Work out the finished part from the listing and answer in its coordinate system (mm). A direction names the side the tool comes from. Coordinates: 2 decimals unless noted, no trailing zeros. Order: outer loops, then holes, each group sorted by start corner. A loop starts at its lowest first (then second) coordinate and runs counter-clockwise, first axis right, second up. Notation, with made-up numbers: M 77,8 L 98,8 A28 cw 98,28 Z; hole C 15,55 d8. An arc over 180 degrees is marked long. Use a Markdown table: item, result.
from build123d import *

# Parameters (mm, degrees)
CROQUIS1_W              = 250
CROQUIS1_H              = 100
SALIENTE_EXTRUIR1_DEPTH = 240
CROQUIS1_3_W            = 250
CROQUIS1_3_H            = 100
SALIENTE_EXTRUIR2_DEPTH = 10
REDONDEO2_R             = 60
CROQUIS7_RX             = 76.972297538
CROQUIS7_RY             = 67.204239475
CORTAR_EXTRUIR4_DEPTH   = 143
CROQUIS8_RX             = 76.972297538
CROQUIS8_RY             = 67.204239475
SALIENTE_EXTRUIR3_DEPTH = 5
CROQUIS10_W             = 80
CROQUIS10_H             = 10
SALIENTE_EXTRUIR4_DEPTH = 140
CROQUIS10_4_W           = 60
CROQUIS10_4_H           = 40
SALIENTE_EXTRUIR5_DEPTH = 5
CROQUIS10_7_W           = 10
CROQUIS10_7_H           = 40
SALIENTE_EXTRUIR6_DEPTH = 40
REDONDEO3_R             = 10


with BuildPart() as part:
    # Croquis1 → Saliente-Extruir1 (new body)
    with BuildSketch(Plane(origin=(0, 0, 0), x_dir=(1, 0, 0), z_dir=(0, 1, 0))):
        with Locations((125, 50)):
            Rectangle(CROQUIS1_W, CROQUIS1_H)
    extrude(amount=SALIENTE_EXTRUIR1_DEPTH)

    # Croquis1_3 → Saliente-Extruir2 (add)
    with BuildSketch(Plane(origin=(0, 0, 0), x_dir=(1, 0, 0), z_dir=(0, 1, 0))):
        with Locations((125, 150)):
            Rectangle(CROQUIS1_3_W, CROQUIS1_3_H)
    extrude(amount=SALIENTE_EXTRUIR2_DEPTH)

    # Redondeo2
    redondeo2_edges = [part.edges().sort_by_distance(p)[0] for p in [
        (250, 240, -50),
        (0, 240, -50),
    ]]
    fillet(redondeo2_edges, radius=REDONDEO2_R)

    # Croquis7 → Cortar-Extruir4 (cut)
    with BuildSketch(Plane.XY):
        with Locations(Location((125, 120), (0, 0, 90))):
            Ellipse(CROQUIS7_RX, CROQUIS7_RY)
    extrude(amount=-CORTAR_EXTRUIR4_DEPTH, mode=Mode.SUBTRACT)

    # Croquis8 → Saliente-Extruir3 (add)
    with BuildSketch(Plane.XY):
        with BuildLine():
            add(Edge.make_bspline(
                [(125, 33.027702462), (127.716922997, 33.027702462), (130.404614336, 33.188438016), (135.724227666, 33.816566957), (138.356140016, 34.284013351), (143.564938997, 35.521474998), (146.141826175, 36.291487238), (149.32789788, 37.44666128), (149.963373673, 37.687404872), (151.222655871, 38.185011316), (151.847502015, 38.442239729), (153.70789977, 39.238771481), (154.929321189, 39.80290291), (158.538604748, 41.591903506), (160.871628277, 42.913129324), (165.395861295, 45.804761696), (167.58815404, 47.376066564), (171.826538699, 50.764218527), (173.840461698, 52.555062734), (177.671334874, 56.317817281), (179.488232347, 58.289776068), (182.931848653, 62.408514262), (184.558548159, 64.555311436), (186.856901598, 67.905760262), (187.596747198, 69.04071402), (189.017296342, 71.333449758), (189.6993083, 72.493124445), (192.971944449, 78.356200717), (195.154024171, 83.251956302), (197.358832322, 89.617795434), (197.773446154, 90.903439911), (198.549527035, 93.499465527), (198.90845874, 94.801347136), (199.900213511, 98.718294557), (200.448185039, 101.344637868), (201.763342829, 109.267362405), (202.204539447, 114.607070459), (202.204164292, 121.355053919), (202.176088659, 122.711265866), (202.064301478, 125.410452751), (201.980723301, 126.754629699), (201.648104971, 130.771139961), (201.317354659, 133.427486666), (200.000943496, 141.333104769), (198.694169349, 146.519550286), (196.490505918, 152.89104827), (196.019747164, 154.162853647), (195.025553036, 156.678150817), (194.502863938, 157.920234824), (192.858566532, 161.600125171), (191.660898436, 163.991673425), (187.761672007, 170.980079827), (184.75725411, 175.392744669), (180.875974654, 180.052106022), (180.437687128, 180.565534743), (179.546751621, 181.583658434), (179.09337423, 182.089135096), (177.717535309, 183.585353779), (176.779803074, 184.555633176), (173.905444326, 187.385345487), (171.907805387, 189.163850968), (167.748045081, 192.502690959), (165.585944795, 194.06305343), (161.090554052, 196.95671019), (158.757317239, 198.290075632), (155.72577479, 199.804250133), (155.112808717, 200.099822067), (153.88335661, 200.671549412), (153.266110917, 200.948114377), (151.406864587, 201.750096433), (150.157359681, 202.247819081), (146.379036893, 203.630980583), (143.820490433, 204.406706354), (138.623300542, 205.662560658), (135.98466882, 206.142732406), (132.634166248, 206.550255722), (131.96144789, 206.622099252), (130.610691005, 206.746152274), (129.93172719, 206.798392098), (127.900475049, 206.924426335), (126.55019563, 206.968001148), (122.510773219, 206.97998383), (119.833015326, 206.829969745), (114.507334656, 206.219611994), (111.859412215, 205.759264851), (107.910237087, 204.832541616), (106.593459447, 204.482838697), (103.994656921, 203.711410555), (102.711704261, 203.289784981), (98.91073308, 201.920359147), (96.440473583, 200.868288733), (91.623019608, 198.495465534), (89.275838057, 197.174684523), (85.847080779, 194.992620648), (84.71874619, 194.230876818), (82.517429794, 192.658127473), (81.441211058, 191.845169128), (78.283535549, 189.32908586), (76.27287878, 187.548949253), (72.432879578, 183.791453982), (70.603560889, 181.814069491), (67.99406522, 178.7017115), (67.145842384, 177.638458972), (65.509882594, 175.484104304), (64.72007818, 174.390671655), (62.432585129, 171.063111394), (61.016620532, 168.781834632), (58.394106502, 164.098462965), (57.187582612, 161.696353323), (55.532932124, 158.003686436), (55.007282323, 156.757854747), (54.007986074, 154.236189011), (53.536955939, 152.966840124), (51.326504906, 146.593244825), (50.011292376, 141.394042449), (48.68568488, 133.451947581), (48.35242998, 130.780535642), (48.017922664, 126.736804027), (47.934071147, 125.381056898), (47.82305979, 122.680583454), (47.7956054, 121.333200704), (47.79638432, 114.610332415), (48.235235275, 109.276623608), (49.552019564, 101.343057777), (50.101380969, 98.70977145), (51.097892129, 94.777389169), (51.459613379, 93.467418163), (52.234572443, 90.878122589), (52.64839956, 89.596085706), (54.84833069, 83.248504751), (57.023259968, 78.369066466), (60.932315801, 71.359424739), (62.343788817, 69.074787684), (64.633950857, 65.730613408), (65.428738625, 64.626504273), (67.06308957, 62.467122017), (67.902663487, 61.411404642), (70.488298836, 58.315872226), (72.301112731, 56.347504426), (76.107190252, 52.603909795), (78.100429201, 50.828656551), (82.275122661, 47.479603046), (84.456517338, 45.90573874), (87.309903664, 44.073958286), (87.887913061, 43.71382706), (89.049899878, 43.011672104), (89.634271423, 42.669355361), (91.39746439, 41.668541908), (92.5863576, 41.036165001), (96.193121975, 39.24298859), (98.65097198, 38.185868736), (103.674761223, 36.35194367), (106.240682844, 35.57509277), (110.174376905, 34.629763782), (111.499773132, 34.351388781), (114.179927084, 33.870783809), (115.524400715, 33.670430265), (118.219575281, 33.349651967), (119.570693495, 33.229152241), (121.602683565, 33.108421489), (122.280899507, 33.078186262), (123.639111575, 33.03782677), (124.320769251, 33.027702462), (125, 33.027702462)],
                knots=[0, 0, 0, 0, 0.015625, 0.015625, 0.03125, 0.03125, 0.046875, 0.046875, 0.05078125, 0.05078125, 0.0546875, 0.0546875, 0.0625, 0.0625, 0.078125, 0.078125, 0.09375, 0.09375, 0.109375, 0.109375, 0.125, 0.125, 0.140625, 0.140625, 0.1484375, 0.1484375, 0.15625, 0.15625, 0.1875, 0.1875, 0.1953125, 0.1953125, 0.203125, 0.203125, 0.21875, 0.21875, 0.25, 0.25, 0.2578125, 0.2578125, 0.265625, 0.265625, 0.28125, 0.28125, 0.3125, 0.3125, 0.3203125, 0.3203125, 0.328125, 0.328125, 0.34375, 0.34375, 0.375, 0.375, 0.37890625, 0.37890625, 0.3828125, 0.3828125, 0.390625, 0.390625, 0.40625, 0.40625, 0.421875, 0.421875, 0.4375, 0.4375, 0.44140625, 0.44140625, 0.4453125, 0.4453125, 0.453125, 0.453125, 0.46875, 0.46875, 0.484375, 0.484375, 0.48828125, 0.48828125, 0.4921875, 0.4921875, 0.5, 0.5, 0.515625, 0.515625, 0.53125, 0.53125, 0.5390625, 0.5390625, 0.546875, 0.546875, 0.5625, 0.5625, 0.578125, 0.578125, 0.5859375, 0.5859375, 0.59375, 0.59375, 0.609375, 0.609375, 0.625, 0.625, 0.6328125, 0.6328125, 0.640625, 0.640625, 0.65625, 0.65625, 0.671875, 0.671875, 0.6796875, 0.6796875, 0.6875, 0.6875, 0.71875, 0.71875, 0.734375, 0.734375, 0.7421875, 0.7421875, 0.75, 0.75, 0.78125, 0.78125, 0.796875, 0.796875, 0.8046875, 0.8046875, 0.8125, 0.8125, 0.84375, 0.84375, 0.859375, 0.859375, 0.8671875, 0.8671875, 0.875, 0.875, 0.890625, 0.890625, 0.90625, 0.90625, 0.921875, 0.921875, 0.92578125, 0.92578125, 0.9296875, 0.9296875, 0.9375, 0.9375, 0.953125, 0.953125, 0.96875, 0.96875, 0.9765625, 0.9765625, 0.984375, 0.984375, 0.9921875, 0.9921875, 0.99609375, 0.99609375, 1, 1, 1, 1], degree=3))
        make_face()
        with Locations(Location((125, 120), (0, 0, 90))):
            Ellipse(CROQUIS8_RX, CROQUIS8_RY, mode=Mode.SUBTRACT)
    extrude(amount=SALIENTE_EXTRUIR3_DEPTH)

    # Croquis10 → Saliente-Extruir4 (add)
    with BuildSketch(Plane(origin=(0, 240, 0), x_dir=(1, 0, 0), z_dir=(0, 1, 0))):
        with Locations((125, 75)):
            Rectangle(CROQUIS10_W, CROQUIS10_H)
    extrude(amount=SALIENTE_EXTRUIR4_DEPTH)

    # Croquis10_4 → Saliente-Extruir5 (add)
    with BuildSketch(Plane(origin=(0, 240, 0), x_dir=(1, 0, 0), z_dir=(0, 1, 0))):
        with Locations((125, 50)):
            Rectangle(CROQUIS10_4_W, CROQUIS10_4_H)
    extrude(amount=SALIENTE_EXTRUIR5_DEPTH)

    # Croquis10_7 → Saliente-Extruir6 (add)
    with BuildSketch(Plane(origin=(0, 240, 0), x_dir=(1, 0, 0), z_dir=(0, 1, 0))):
        with Locations((160, 50)):
            Rectangle(CROQUIS10_7_W, CROQUIS10_7_H)
        with Locations((90, 50)):
            Rectangle(CROQUIS10_7_W, CROQUIS10_7_H)
    extrude(amount=SALIENTE_EXTRUIR6_DEPTH)

    # Redondeo3
    redondeo3_edges = [part.edges().sort_by_distance(p)[0] for p in [
        (165, 380, -75),
        (85, 380, -75),
        (160, 280, -30),
        (90, 280, -30),
    ]]
    fillet(redondeo3_edges, radius=REDONDEO3_R)


solid = part.part
(1) A cutting plane is placed at B-B (x = 39.5). Determine the outline of the cut face in (y, z), then the cut area to 3 significant figures.
Conclusion:
| item | result |
|---|---|
| outline | M 0,-200 L 10,-200 L 10,-100 L 236.39,-100 L 236.39,0 L 0,0 Z |
| area | 24,600 mm2 |
(2) Which of the six approach directions +Z, -Z, +X, -X, +Y, -Y give full straight-line access (tool end or side, diameter ignored) to faces 5 (the flat face through (123, 10, -151)), 6 (the flat face through (155, 262, -50)), 7 (the flat face through (165, 275, -60)), 8 (the flat face through (95, 38, 0)), 9 (the flat face through (160, 280, -55))?
Conclusion:
| item | result |
|---|---|
| face 5 | -Z, +X, -X, +Y |
| face 6 | +Z, +Y |
| face 7 | +Z, -Z, +X, +Y |
| face 8 | +Z |
| face 9 | +Z, +X, -X, +Y |
(3) A cutting plane is placed at A-A (y = 254). Determine the outline of the cut face in (x, z).
Conclusion:
| item | result |
|---|---|
| outline | M 85,-80 L 165,-80 L 165,-30 L 155,-30 L 155,-70 L 95,-70 L 95,-30 L 85,-30 Z |
(4) Given P1, Ø24, axis at x = 122.5, y = 254, coming from the +Z side; P2, Ø17.5, axis at y = 254, z = -50, coming from the -X side; P3, Ø8, axis at x = 189.5, z = -53, coming from the +Y side, each flat-ended and moving along its own axis, determine where each tip first touches the part or whether it passes through.
Conclusion:
| item | result |
|---|---|
| P1 | z = -30 |
| P2 | x = 85 |
| P3 | y = 240 |
(5) A cutting plane is placed at D-D (x = 234.5). Determine the outline of the cut face in (y, z), then the cut area to 3 significant figures.
Conclusion:
| item | result |
|---|---|
| outline | M 0,-200 L 10,-200 L 10,-100 L 220.25,-100 L 220.25,0 L 0,0 Z |
| area | 23,000 mm2 |
(6) Straight lines are drawn through the part: L1, parallel to Z at x = 27, y = 84; L2, parallel to Z at x = 154, y = 333.5; L3, parallel to X at y = 249, z = -46.5. For each, find the intervals that lie inside material, in ascending order.
Conclusion:
| item | result |
|---|---|
| L1 | -100 to 0 |
| L2 | -80 to -70 |
| L3 | 85 to 95, 155 to 165 |
(7) Determine the mould class of faces 1 (the cylindrical face through (161.99, 377.15, -75.07)), 2 (the flat face through (125, 245, -50)), 3 (the flat face through (90, 280, -55)), 4 (the flat face through (85, 275, -60)) for opening direction X: pulls with the +X half, pulls with the -X half, needs draft (parallel to the pull), parting line crosses it, or undercut.
Conclusion:
| item | result |
|---|---|
| face 1 | pulls with the +X half |
| face 2 | undercut |
| face 3 | needs draft |
| face 4 | pulls with the -X half |
(8) A cutting plane is placed at C-C (z = -115.5). Determine the outline of the cut face in (x, y).
Conclusion:
| item | result |
|---|---|
| outline | M 0,0 L 250,0 L 250,10 L 0,10 Z |
